Work out the finished part from the listing and answer in its coordinate system (mm). A direction names the side the tool comes from. Give positions to 0.01 mm unless a question says otherwise; leave off trailing zeros. Order: outer loops, then holes, each group sorted by start corner. A loop starts at its lowest first (then second) coordinate and runs counter-clockwise, first axis right, second up. Notation, with made-up numbers: (33, 17.25) - (56, 17.25) arc R15 ccw to (56, 32.25) - close; hole circle Ø5 at (1, 22). An arc over 180 degrees is marked (long way). Write each question's results on one line, items separated by ' | '.
from build123d import *

# Parameters (mm, degrees)
F2_W            = 3
F2_H            = 3
F3_DEPTH        = 19
F5_R            = 9.49999
F6_R            = 5
F7_R            = 2
F8_R            = 1
F9_SIZE         = 2.99999
F10_D           = 3.7973
F10_CSINK_D     = 7.7978
F10_CSINK_ANGLE = 82
F11_R           = 2.9999


# Not quite as in the source:
# - a fillet or chamfer is up to 0.001 mm smaller than in the source, because OpenCascade refuses the exact size


with BuildPart() as f3:
    # F2 (on Top) → F3 (new body)
    with BuildSketch(Plane.XY):
        with BuildLine():
            Line((35.5, -27.8585158202), (-35.5, -27.8585158202))
            Line((-35.5, -27.8585158202), (-35.5, -30.8585158202))
            Line((-35.5, -30.8585158202), (35.5, -30.8585158202))
            ThreePointArc((35.5, -30.8585158202), (41.1568542495, -28.5153700696), (43.5, -22.8585158202))
            Line((43.5, -22.8585158202), (43.5, -22.3585158202))
            ThreePointArc((43.5, -22.3585158202), (41.1568542495, -16.7016615707), (35.5, -14.3585158202))
            Line((35.5, -14.3585158202), (-6.5, -14.3585158202))
            Line((-6.5, -14.3585158202), (-6.5, -16.3585158202))
            Line((-6.5, -16.3585158202), (-6.5, -17.3585158202))
            Line((-6.5, -17.3585158202), (-3.5, -17.3585158202))
            Line((-3.5, -17.3585158202), (35.5, -17.3585158202))
            ThreePointArc((35.5, -17.3585158202), (39.0355339059, -18.8229819142), (40.5, -22.3585158202))
            Line((40.5, -22.3585158202), (40.5, -22.8585158202))
            ThreePointArc((40.5, -22.8585158202), (39.0355339059, -26.3940497261), (35.5, -27.8585158202))
        make_face()
        with Locations((-2, -25.8585158202)):
            Rectangle(F2_W, F2_H)
        Polygon((-3.5, -24.3585158202), (-3.5, -17.3585158202), (-6.5, -17.3585158202), (-6.5, -27.3585158202), (-3.5, -27.3585158202), align=None)
        Polygon((-9.5, -17.3585158202), (-6.5, -17.3585158202), (-6.5, -16.3585158202), (-6.5, -14.3585158202), (-9.5, -14.3585158202), align=None)
    extrude(amount=F3_DEPTH)

    # F5 (radius 9.5 in the source; OpenCascade refuses exactly that, so slightly less here)
    f5_edges = [f3.edges().sort_by_distance(p)[0] for p in [
        (-35.5, -29.358516, 19),
        (-35.5, -29.358516, 0),
    ]]
    fillet(f5_edges, radius=F5_R)

    # F6
    f6_edges = [f3.edges().sort_by_distance(p)[0] for p in [
        (-9.5, -15.858516, 19),
        (-9.5, -15.858516, 0),
    ]]
    fillet(f6_edges, radius=F6_R)

    # F7
    f7_edges = [f3.edges().sort_by_distance(p)[0] for p in [
        (15.5, -14.358516, 0),
    ]]
    fillet(f7_edges, radius=F7_R)

    # F8
    f8_edges = [f3.edges().sort_by_distance(p)[0] for p in [
        (-3.5, -24.358516, 9.5),
    ]]
    fillet(f8_edges, radius=F8_R)

    # F9 (size 3 in the source; OpenCascade refuses exactly that, so slightly less here)
    f9_edges = [f3.edges().sort_by_distance(p)[0] for p in [
        (-6.5, -17.358516, 9.5),
    ]]
    chamfer(f9_edges, length=F9_SIZE)

    # F10 (through all)
    with Locations(Plane(origin=(0, -27.8585158202, 0), x_dir=(-1, 0, 0), z_dir=(0, 1, 0))):
        with Locations((25.5, 9.5)):
            CounterSinkHole(F10_D / 2, F10_CSINK_D / 2, counter_sink_angle=F10_CSINK_ANGLE)

    # F11 (radius 3 in the source; OpenCascade refuses exactly that, so slightly less here)
    f11_edges = [f3.edges().sort_by_distance(p)[0] for p in [
        (-0.5, -24.358516, 9.5),
        (-6.5, -27.358516, 9.5),
    ]]
    fillet(f11_edges, radius=F11_R)


solid = f3.part
1. A tool of negligible diameter and unlimited length cuts with its end or side. For faces 4 (the face through (-6.563, -19.442, 18.554)), 5 (the face through (-3.5, -20, 9)), 6 (the face through (0, -27.859, 9)), 7 (the face through (10.1, -28.1, 19)), from which of +Z, -Z, +X, -X, +Y, -Y can it reach the whole face along a straight path? Write none if from no direction.
Answer list:
face 4: +Z, -X, +Y | face 5: +Z, -Z | face 6: +Z, -Z, -X | face 7: +Z, +X, -X, +Y, -Y
2. Given P1, Ø8, axis at y = -17.5, z = 15, coming from the -X side; P2, Ø2, axis at x = -15, z = 16, coming from the +Y side; P3, Ø1.8, axis at y = -21, z = 11.5, coming from the +X side, each flat-ended and moving along its own axis, determine where each tip first touches the part or whether it passes through.
Answer list:
P1: x = -9.5 | P2: y = -27.86 | P3: x = 43.49
3. Straight lines are drawn through the part: line 1 (Y direction, x = 7, z = 12); line 2 (Z direction, x = 18.5, y = -29); line 3 (X direction, y = -30, z = 7.75). For each, find the intervals that lie inside material, in ascending order. Write a range as [from, to].
Answer list:
line 1: [-30.86, -27.86], [-17.36, -14.36] | line 2: [0.01, 18.99] | line 3: [-34.97, -26.54], [-24.46, 39.11]
4. A cutting plane is placed at A-A, the plane x = 6. Write down the section's boundary in (y, z).
Answer list:
outline: (-30.86, 2) arc R2 ccw to (-28.86, 0) - (-27.86, 0) - (-27.86, 19) - (-28.86, 19) arc R2 ccw to (-30.86, 17) - close; (-17.36, 0) - (-16.36, 0) arc R2 ccw to (-14.36, 2) - (-14.36, 17) arc R2 ccw to (-16.36, 19) - (-17.36, 19) - close
5. Determine the mould class of faces 1 (the face through (-2, -27.359, 9)), 2 (the face through (42.9, -22.61, 0.57)), 3 (the face through (4.319, -30.257, 18.43)) for opening direction Y: +Y half, -Y half, draft (parallel to the pull), parting line (faces both ways), or undercut.
Answer list:
face 1: undercut | face 2: draft | face 3: -Y half
